Verification items for the finished model (mm, model axes). Coordinates: 2 decimals unless noted, no trailing zeros. Write each loop counter-clockwise with the first axis right and the second up, starting at its lowest first coordinate (ties: lowest second). Pieces come first, ordered by that corner, then holes. Notation, with made-up numbers: (-1.75, 56) -> (51.25, 56) arc R32 ccw to (51.25, 82) -> close; hole circle Ø7 at (-6.5, 27). An arc over 180 degrees is marked (long way). Answer in a Markdown table with one row per item.
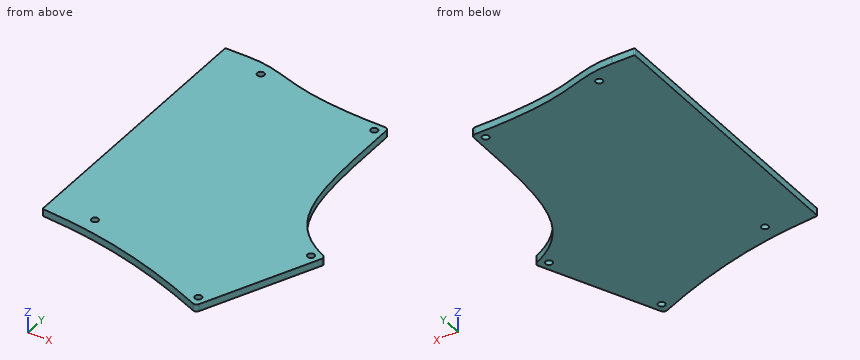
```python
from build123d import *

# Parameters (mm, degrees)
PAD010_DEPTH    = 3
SKETCH045_R     = 1.45
POCKET015_DEPTH = 30
FILLET008_R     = 1.5
FILLET016_R     = 0.5


with BuildPart() as part:
    # Sketch034 → Pad010 (new body)
    with BuildSketch(Plane.XY):
        with BuildLine():
            add(Edge.make_bspline(
                [(76.2, -18.332251), (89.391212, -19.369368), (115.462334, -21.271145), (153.231854, -38.154949)],
                knots=[0, 0, 0, 0, 1, 1, 1, 1], degree=3))
            Line((153.231854, -38.154949), (175.310198, 11.234895))
            add(Edge.make_bspline(
                [(150.875, 88.9625), (150.875, 42.8625), (150.875, 22.157965), (175.310198, 11.234895)],
                knots=[0, 0, 0, 0, 1, 1, 1, 1], degree=3))
            add(Edge.make_bspline(
                [(85.725, 98.4875), (104.775, 98.4875), (104.775, 88.9625), (150.875, 88.9625)],
                knots=[0, 0, 0, 0, 1, 1, 1, 1], degree=3))
            Line((85.725, 98.4875), (76.2, 98.4875))
            Line((76.2, 98.4875), (76.2, -18.332251))
        make_face()
    extrude(amount=PAD010_DEPTH)

    # Sketch045 → Pocket015 (cut)
    with BuildSketch(Plane.XY):
        with Locations((-4.375, -4.375)):
            Circle(SKETCH045_R)
        with Locations((-4.375, 80.575)):
            Circle(SKETCH045_R)
        with Locations((151.401832, -33.366184)):
            Circle(SKETCH045_R)
        with Locations((170.521433, 9.404873)):
            Circle(SKETCH045_R)
        with Locations((147.25, 85.3375)):
            Circle(SKETCH045_R)
        with Locations((43.25, -13.9)):
            Circle(SKETCH045_R)
        with Locations((57.15, 92.085)):
            Circle(SKETCH045_R)
        with Locations((95.25, 92.085)):
            Circle(SKETCH045_R)
        with Locations((95.25, -13.9)):
            Circle(SKETCH045_R)
    extrude(amount=POCKET015_DEPTH, mode=Mode.SUBTRACT)

    # Fillet008
    fillet008_edges = [part.edges().sort_by_distance(p)[0] for p in [
        (150.875, 88.9625, 1.5),
        (175.310198, 11.234895, 1.5),
        (153.231854, -38.154949, 1.5),
    ]]
    fillet(fillet008_edges, radius=FILLET008_R)

    # Fillet016
    fillet016_edges = [part.edges().sort_by_distance(p)[0] for p in [
        (76.2, 98.4875, 1.5),
        (76.2, -18.332251, 1.5),
    ]]
    fillet(fillet016_edges, radius=FILLET016_R)


with BuildPart() as part_1:
    # Body009 placement: moved
    add(part.part.moved(Location((0, 0, -18))))


solid = part_1.part
```
1. Go/stop test with flat-tipped pins: pin 1 (2.5 mm diameter, centred on x = 95.25, y = -13.9, fed in from +Z); pin 2 (4.5 mm diameter, centred on x = 151.4, y = -33.37, fed in from +Z). Record where each tip stops, or that it passes through.
Findings below:
| item | result |
|---|---|
| pin 1 | passes through |
| pin 2 | stops at z = -15 |
2. Sectioned sample at B-B, the plane z = -15.8. Count the separate pieces of the cut face and the enclosed holes in it, and give its area (3 significant figures).
Findings below:
| item | result |
|---|---|
| separate pieces | 1 |
| enclosed holes | 5 |
| area | 9,780 mm² |
3. Sectioned sample at A-A, the plane y = -13.9. Record the cut outline in (x, z).
Findings below:
| item | result |
|---|---|
| outline | (76.2, -18) -> (93.8, -18) -> (93.8, -15) -> (76.2, -15) -> close; (96.7, -18) -> (164.07, -18) -> (164.07, -15) -> (96.7, -15) -> close |
4. Sectioned sample at D-D, the plane y = 6. Record the cut outline in (x, z).
Findings below:
| item | result |
|---|---|
| outline | (76.2, -18) -> (172.97, -18) -> (172.97, -15) -> (76.2, -15) -> close |
5. Material ranges on probe 1 along Y at (x, z) = (95, -16.4); probe 2 along X at (y, z) = (80, -16.85); probe 3 along Y at (x, z) = (95.5, -17.2), recorded low to high. Write a range as from..to.
Findings below:
| item | result |
|---|---|
| probe 1 | y = -20.39..-15.33, -12.47..90.66, 93.51..97.58 |
| probe 2 | x = 76.2..150.88 |
| probe 3 | y = -20.46..-15.33, -12.47..90.66, 93.51..97.47 |
